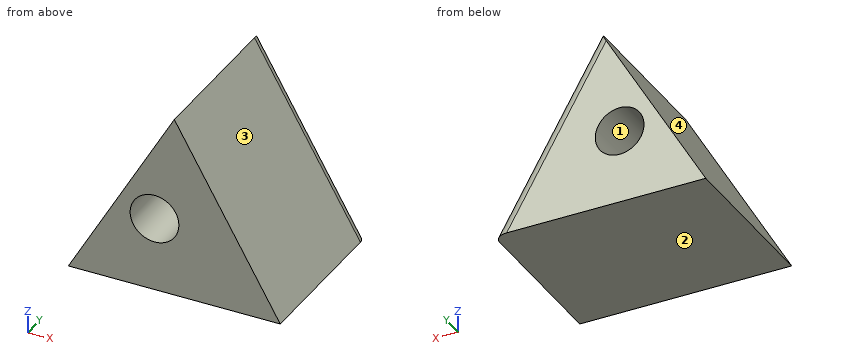
from build123d import *

# Parameters (mm, degrees)
F1_DEPTH = 98
F2_R     = 6.518377
F3_R     = 14.415035
F4_DEPTH = 98.001


with BuildPart() as f1:
    # F0 (on Front) → F1 (new body)
    with BuildSketch(Plane.XZ):
        Polygon((-62.669813, -36.182433), (62.669813, -36.182433), (0, 72.364867), align=None)
    extrude(amount=F1_DEPTH)

    # F2
    f2_edges = [f1.edges().sort_by_distance(p)[0] for p in [
        (31.334906, 0, 18.091217),
    ]]
    fillet(f2_edges, radius=F2_R)

    # F3 (on face) → F4 (cut, through all)
    with BuildSketch(Plane.XZ.offset(98)):
        with Locations((-11.717295, 7.68878)):
            Circle(F3_R)
    extrude(amount=-F4_DEPTH, mode=Mode.SUBTRACT)


solid = f1.part
Design review of the part built by this model. Coordinates are the model's own, in mm. Face numbers are marked on the shaded views. Coordinates: 2 decimals unless noted, no trailing zeros. Write each loop counter-clockwise with the first axis right and the second up, starting at its lowest first coordinate (ties: lowest second). Pieces come first, ordered by that corner, then holes. Notation, with made-up numbers: (11.5, -22.75) - (59.5, -22.75) arc R31 ccw to (59.5, 3.25) - close; hole circle Ø6 at (8.25, 75). An arc over 180 degrees is marked (long way). One line per item, written item: value.
1) Add section C-C (x = -44.5). State the section outline as (y, z) points, plus the area to 3 significant figures.
Answer sheet:
outline: (-98, -36.18) - (0, -36.18) - (0, -4.71) - (-98, -4.71) - close
area: 3,080 mm2
2) Insertion check: pin 1 (8 mm diameter, centred on x = 41.5, y = -37, fed in from +Z); pin 2 (4 mm diameter, centred on x = 28, y = -73.5, fed in from +Z); pin 3 (1 mm diameter, centred on y = -36, z = 31, fed in from -X). Each pin has a flat end and moves straight along its axis. Give the tip position at first contact, or say it passes through.
Answer sheet:
pin 1: stops at z = 7.41
pin 2: stops at z = 27.33
pin 3: stops at x = -24.17
3) Mouldability with a two-part tool opening along X and no side actions: class the marked faces 1, 2, 3 and 4 as +X half, -X half, draft (parallel to the pull), parting line (faces both ways), or undercut.
Answer sheet:
face 1: undercut
face 2: draft
face 3: +X half
face 4: -X half
4) Add section B-B (y = -20). State the section outline as (x, z) points, plus the area to 3 significant figures.
Answer sheet:
outline: (-62.67, -36.18) - (62.67, -36.18) - (0, 72.36) - close; hole circle Ø28.83 at (-11.72, 7.69)
area: 6,150 mm2
5) Add section A-A (x = -18.5). State the section outline as (y, z) points, plus the area to 3 significant figures.
Answer sheet:
outline: (-98, -36.18) - (0, -36.18) - (0, -5.03) - (-98, -5.03) - close; (-98, 20.41) - (0, 20.41) - (0, 40.32) - (-98, 40.32) - close
area: 5,000 mm2
6) To check wall thickness, follow probe 1 along X at (y, z) = (-11, 13); probe 2 along X at (y, z) = (-25, 6.5); probe 3 along Z at (x, y) = (-7, -77). State the ranges of each line that lie inside material, in increasing order.
Answer sheet:
probe 1: x = -34.27 to -25.12, 1.68 to 34.27
probe 2: x = -38.03 to -26.08, 2.65 to 38.03
probe 3: z = -36.18 to -5.93, 21.31 to 60.24
